The model under review builds one solid part; all positions refer to its coordinate system, in mm. A direction names the side the tool comes from. Coordinates: 2 decimals unless noted, no trailing zeros. Loops run counter-clockwise (first coordinate to the right, second up) from the corner with the lowest first, then second, coordinate; pieces in that order, holes last. Notation, with made-up numbers: (32, -38) - (85, -38) arc R20 ccw to (85, -1) - close; hole circle Ø6 at (76.5, 45). An arc over 180 degrees is marked (long way). Use a Markdown table: item, result. Add a question column.
1) Add section C-C, the plane z = 2.75. Give the boundary of the cut face in (x, y).
2) The part is to be moulded in two halves that separate along Z. For faces 5 (the cylindrical face through (-44.461, -49.689, 0.285)), 6 (the cylindrical face through (-64.73, -61.99, 6.92)), 7 (the cylindrical face through (-58.914, -37.391, 13.715)), 8 (the cylindrical face through (-59.81, -40.74, 7.6)), say which applies: pulls with the +Z half, pulls with the -Z half, needs draft (parallel to the pull), parting line crosses it, or undercut.
3) Add section A-A, the plane y = -55. Give the boundary of the cut face in (x, z), and give its area (3 significant figures).
4) To check wall thickness, follow L1, parallel to Y at x = -50, z = 7.25; L2, parallel to X at y = -42, z = 9.5; L3, parallel to Y at x = -66.5, z = 6.5. State the ranges of each line that lie inside material, in increasing order. Write a range as [from, to].
5) Add section B-B, the plane x = -38. Give the boundary of the cut face in (y, z).
6) Clearance check with flat-ended pins moving along their axes: pin 1 (1 mm diameter, centred on y = -51.5, z = 9, fed in from -X); pin 2 (7 mm diameter, centred on y = -41, z = 10, fed in from +X); pin 3 (8 mm diameter, centred on x = -38.66, z = 7, fed in from +Y). State where each tip first meets the part, or that it passes through.
7) For faces 1 (the cylindrical face through (-43.56, -62.02, 6.92)), 2 (the flat face through (-70, -62.59, 4)), 3 (the cylindrical face through (-38.709, -62.891, 13.715)), 4 (the cylindrical face through (-38.709, -62.891, 0.285)), list the 3-axis set-ups (+Z, -Z, +X, -X, +Y, -Y) from which the entire face can be reached by the end or side of a thin tool; tool diameter is ignored.
8) Add section D-D, the plane z = 8.5. Give the number of separate pieces and of enclosed holes in the cut face, and give its area (3 significant figures).
```python
from build123d import *

# Parameters (mm, degrees)
F1_DEPTH = 14
F2_R     = 3.5
F2_R_2   = 2
F3_DEPTH = 5
F4_DEPTH = 25
F5_R     = 2.5
F6_DEPTH = 25
F7_R     = 1


with BuildPart() as f1:
    # F0 (on Top) → F1 (new body)
    with BuildSketch(Plane.XY):
        with BuildLine():
            Line((-75.1601234078, -64.5899677277), (-75.1601234078, -74.5899677277))
            Line((-75.1601234078, -74.5899677277), (-33.1601234078, -74.5899677277))
            Line((-33.1601234078, -74.5899677277), (-33.1601234078, -64.5899677277))
            ThreePointArc((-33.1601234078, -64.5899677277), (-33.7459098455, -63.1757541653), (-35.1601234078, -62.5899677277))
            Line((-35.1601234078, -62.5899677277), (-42.1601234078, -62.5899677277))
            ThreePointArc((-42.1601234078, -62.5899677277), (-43.5743369702, -62.00418129), (-44.1601234078, -60.5899677277))
            Line((-44.1601234078, -60.5899677277), (-44.1601234078, -39.0899677277))
            ThreePointArc((-44.1601234078, -39.0899677277), (-44.7459098455, -37.6757541653), (-46.1601234078, -37.0899677277))
            Line((-46.1601234078, -37.0899677277), (-52.5748137326, -37.0899677277))
            Line((-52.5748137326, -37.0899677277), (-52.5748137326, -45.8031902796))
            ThreePointArc((-52.5748137326, -45.8031902796), (-49.3898059105, -47.9507272885), (-48.1601234078, -51.5899677277))
            ThreePointArc((-48.1601234078, -51.5899677277), (-57.8690220349, -56.3063297763), (-55.5748137326, -45.7591314853))
            Line((-55.5748137326, -45.7591314853), (-55.5748137326, -37.0899677277))
            Line((-55.5748137326, -37.0899677277), (-62.1601234078, -37.0899677277))
            ThreePointArc((-62.1601234078, -37.0899677277), (-63.5743369702, -37.6757541653), (-64.1601234078, -39.0899677277))
            Line((-64.1601234078, -39.0899677277), (-64.1601234078, -60.5899677277))
            ThreePointArc((-64.1601234078, -60.5899677277), (-64.7459098455, -62.00418129), (-66.1601234078, -62.5899677277))
            Line((-66.1601234078, -62.5899677277), (-73.1601234078, -62.5899677277))
            ThreePointArc((-73.1601234078, -62.5899677277), (-74.5743369702, -63.1757541653), (-75.1601234078, -64.5899677277))
        make_face()
    extrude(amount=F1_DEPTH)

    # F2 (on face) → F3 (cut)
    with BuildSketch(Plane.YZ.offset(-44.1601234078)):
        with Locations((-42.6499210298, 7)):
            Circle(F2_R)
        with Locations((-42.6499210298, 7)):
            Circle(F2_R_2, mode=Mode.SUBTRACT)
    extrude(amount=-F3_DEPTH, mode=Mode.SUBTRACT)

    # F4 (cut): a face of the model
    f4_faces = [f1.faces().sort_by_distance(p)[0] for p in [
        (-44.1601234078, -42.6499210298, 7),
    ]]
    extrude(f4_faces, amount=-F4_DEPTH, mode=Mode.SUBTRACT)

    # F5 (on face) → F6 (cut)
    with BuildSketch(Plane(origin=(0, -62.5899677277, 0), x_dir=(-1, 0, 0), z_dir=(0, 1, 0))):
        with Locations((38.6601234078, 7)):
            Circle(F5_R)
        with Locations((69.5535764098, 7)):
            Circle(F5_R)
    extrude(amount=-F6_DEPTH, mode=Mode.SUBTRACT)

    # F7
    f7_edges = [f1.edges().sort_by_distance(p)[0] for p in [
        (-44.160123, -49.839968, 14),
        (-64.160123, -49.839968, 14),
        (-44.160123, -49.839968, 0),
        (-64.160123, -49.839968, 0),
    ]]
    fillet(f7_edges, radius=F7_R)


solid = f1.part
```
From the geometry:
| question | item | result |
|---|---|---|
| 1 | outline | (-75.16, -74.59) - (-33.16, -74.59) - (-33.16, -64.59) arc R2 ccw to (-35.16, -62.59) - (-42.16, -62.59) arc R2 cw to (-44.16, -60.59) - (-44.16, -39.09) arc R2 ccw to (-46.16, -37.09) - (-52.57, -37.09) - (-52.57, -45.8) arc R6 cw (long way) to (-55.57, -45.76) - (-55.57, -37.09) - (-62.16, -37.09) arc R2 ccw to (-64.16, -39.09) - (-64.16, -60.59) arc R2 cw to (-66.16, -62.59) - (-73.16, -62.59) arc R2 ccw to (-75.16, -64.59) - close |
| 2 | face 5 | pulls with the -Z half |
| 2 | face 6 | needs draft |
| 2 | face 7 | pulls with the +Z half |
| 2 | face 8 | undercut |
| 3 | outline | (-64.16, 1) arc R1 ccw to (-63.16, 0) - (-59.1, 0) - (-59.1, 14) - (-63.16, 14) arc R1 ccw to (-64.16, 13) - close; (-49.22, 0) - (-45.16, 0) arc R1 ccw to (-44.16, 1) - (-44.16, 13) arc R1 ccw to (-45.16, 14) - (-49.22, 14) - close |
| 3 | area | 141 mm^2 |
| 4 | L1 | y = [-74.59, -55.91], [-47.27, -44.63], [-40.67, -37.09] |
| 4 | L2 | x = [-64.16, -55.57], [-52.57, -49.16] |
| 4 | L3 | y = [-74.59, -62.59] |
| 5 | outline | (-74.59, 0) - (-63.59, 0) arc R1 ccw to (-62.59, 1) - (-62.59, 4.59) - (-74.59, 4.59) - close; (-74.59, 9.41) - (-62.59, 9.41) - (-62.59, 13) arc R1 ccw to (-63.59, 14) - (-74.59, 14) - close |
| 6 | pin 1 | stops at x = -64.16 |
| 6 | pin 2 | stops at x = -44.16 |
| 6 | pin 3 | stops at y = -62.53 |
| 7 | face 1 | +Z, -Z, +X, +Y |
| 7 | face 2 | +Z, -Z, -X, +Y |
| 7 | face 3 | +Z, +X, +Y |
| 7 | face 4 | -Z, +X, +Y |
| 8 | separate pieces | 5 |
| 8 | enclosed holes | 0 |
| 8 | area | 714 mm^2 |
